from build123d import *

# Parameters (mm, degrees)
ESQUISSE1_W             = 90
ESQUISSE1_H             = 212
BOSS_EXTRU_1_DEPTH      = 2.5
ESQUISSE2_W             = 57
ESQUISSE2_H             = 38.5
BOSS_EXTRU_2_DEPTH      = 2.5
ENL_V_MAT_EXTRU_1_REACH = 172.343
ESQUISSE3_W             = 33.5
ESQUISSE3_H             = 20.5
D_GAGEMENT_M21_D        = 2.4


with BuildPart() as part:
    # Esquisse1 → Boss.-Extru.1 (new body)
    with BuildSketch(Plane.XY):
        Rectangle(ESQUISSE1_W, ESQUISSE1_H)
    extrude(amount=BOSS_EXTRU_1_DEPTH)

    # Esquisse2 → Boss.-Extru.2 (add)
    with BuildSketch(Plane.XY.offset(2.5)):
        Polygon((-75.129202667, 109.181980515), (-45, 79.052777849), (-45, 106), (-17.5, 106), (-47.905591591, 136.405591591), align=None)
        with Locations((-73.5, 0)):
            Rectangle(ESQUISSE2_W, ESQUISSE2_H)
    extrude(amount=-BOSS_EXTRU_2_DEPTH)

    # Esquisse3 → Enlèv. mat.-Extru.1 (cut, up to next)
    with BuildSketch(Plane.XY.offset(2.5), mode=Mode.PRIVATE) as enl_v_mat_extru_1_sk1:
        Polygon((-54.269552622, 130.04163056), (-68.765241636, 115.545941546), (-45.077164466, 91.857864376), (-30.581475452, 106.353553391), align=None)
    enl_v_mat_extru_1_tool1 = extrude(enl_v_mat_extru_1_sk1.sketch, amount=-ENL_V_MAT_EXTRU_1_REACH, mode=Mode.PRIVATE) & part.part
    # Esquisse3 → Enlèv. mat.-Extru.1 (cut, up to next)
    with BuildSketch(Plane.XY.offset(2.5), mode=Mode.PRIVATE) as enl_v_mat_extru_1_sk2:
        with Locations((-85.25, 0)):
            Rectangle(ESQUISSE3_W, ESQUISSE3_H)
    enl_v_mat_extru_1_tool2 = extrude(enl_v_mat_extru_1_sk2.sketch, amount=-ENL_V_MAT_EXTRU_1_REACH, mode=Mode.PRIVATE) & part.part
    add(enl_v_mat_extru_1_tool1.solids().sort_by_distance((-49.673359, 110.949747, 2.5))[0], mode=Mode.SUBTRACT)
    add(enl_v_mat_extru_1_tool2.solids().sort_by_distance((-85.25, 0, 2.5))[0], mode=Mode.SUBTRACT)

    # Dégagement M21 (through all)
    with Locations(Plane.XY.offset(2.5)):
        with Locations((-94.5, -13.5), (-86.5, -13.5), (-78.5, -13.5), (-70.5, -13.5), (-65, -8), (-65, 8), (-70.5, 13.5), (-78.5, 13.5), (-86.5, 13.5), (-94.5, 13.5), (-41.011300474, 90.9739809), (-29.697591975, 102.287689399), (-29.874368671, 109.889087297), (-35.53122292, 115.545941546), (-41.18807717, 121.202795796), (-46.844931419, 126.859650045), (-65.936814511, 107.767766953), (-60.279960262, 102.110912703), (-54.623106012, 96.454058454), (-48.966251763, 90.797204204)):
            Hole(D_GAGEMENT_M21_D / 2)


solid = part.part
For this review, take the finished solid that the model builds, in its own axes (mm). A direction names the side the tool comes from. Round coordinates to 2 decimals unless told otherwise and drop trailing zeros. Write each loop counter-clockwise with the first axis right and the second up, starting at its lowest first coordinate (ties: lowest second). Pieces come first, ordered by that corner, then holes. Notation, with made-up numbers: M 72,25.5 L 129,25.5 A17 cw 129,31.5 Z; hole C 57,-34.75 d2. An arc over 180 degrees is marked long. Write item = value, one per line. Start each with the question number.
(1) For faces 4 (the face through (-51.04, 133.27, 1.27)), 5 (the face through (-42.26, 118.03, 1.27)), list the 3-axis set-ups (+Z, -Z, +X, -X, +Y, -Y) from which the entire face can be reached by the end or side of a thin tool; tool diameter is ignored.
(2) We need section A-A (z = 0.5). Give the number of separate pieces and of enclosed holes in the cut face, then the cut area to 3 significant figures.
(3) Clearance check with flat-ended pins moving along their axes: pin 1 Ø4 at (x, y) = (-78.5, 13.5) entering from +Z; pin 2 Ø1.4 at (x, y) = (-70.5, 13.5) entering from -Z; pin 3 Ø0.8 at (x, z) = (-86.5, 1) entering from -Y; pin 4 Ø1.2 at (y, z) = (42, 1.5) entering from -X. State where each tip first meets the part, or that it passes through.
(4) We need section C-C (x = -14). Give the boundary of the cut face in (y, z).
(5) We need section B-B (y = 54). Give the boundary of the cut face in (x, z).
(6) For line 1 along X through (y, z) = (102, 1.85); line 2 along X through (y, z) = (115, 1.15); line 3 along Y through (x, z) = (-52, 2.25), list the stretches that pass through material, from the lowest coordinate up.
(7) The part is to be moulded in two halves that separate along X. For faces 1 (the face through (-37.931, 99.004, 1.268)), 2 (the face through (-60.28, 94.33, 1.27)), 3 (the face through (-32.5, 121, 1.3)), say which applies: +X half, -X half, draft (parallel to the pull), parting line (faces both ways), or undercut.
Results found:
q1.face_4 = +Z, -Z, -X, +Y
q1.face_5 = +Z, -Z
q2.separate_pieces = 1
q2.enclosed_holes = 20
q2.area = 21,100 mm²
q3.pin_1 = 2.5
q3.pin_2 = through
q3.pin_3 = -19.25
q3.pin_4 = -45
q4.outline = M -106,0 L 106,0 L 106,2.5 L -106,2.5 Z
q5.outline = M -45,0 L 45,0 L 45,2.5 L -45,2.5 Z
q6.line_1 = -67.95 to -61.47, -59.09 to -55.22, -34.94 to -30.86, -28.53 to 45
q6.line_2 = -69.31 to -68.22, -39.23 to -36.6, -34.46 to -26.5
q6.line_3 = -19.25 to 19.25, 86.05 to 98.78, 127.77 to 132.31
q7.face_1 = undercut
q7.face_2 = -X half
q7.face_3 = +X half
